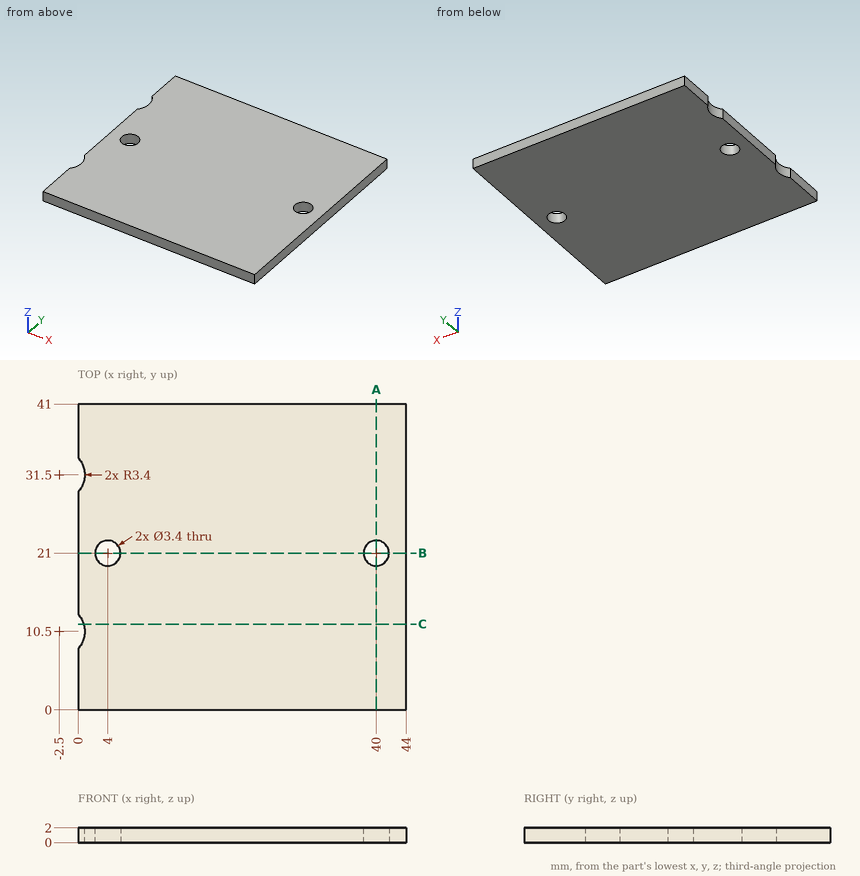
For this review, use the dimensioned drawing (mm, ordinates from the lowest corner) and the shaded views. Give positions to 0.01 mm unless a question says otherwise; leave off trailing zeros. Order: outer loops, then holes, each group sorted by start corner. A loop starts at its lowest first (then second) coordinate and runs counter-clockwise, first axis right, second up.
1. Add section C-C, the plane y = 11.5. State the section outline as (x, z) points.
Solution:
outline: (0.75, 0) - (44, 0) - (44, 2) - (0.75, 2) - close
2. To check wall thickness, follow L1, parallel to Y at x = 40, z = 0.4; L2, parallel to Y at x = 38.5, z = 0.2; L3, parallel to X at y = 33, z = 0.15. State the ranges of each line that lie inside material, in increasing order.
Solution:
L1: y = 0 to 19.3, 22.7 to 41
L2: y = 0 to 20.2, 21.8 to 41
L3: x = 0.55 to 44
3. Add section A-A, the plane x = 40. State the section outline as (y, z) points, then the cut area to 3 significant figures.
Solution:
outline: (0, 0) - (19.3, 0) - (19.3, 2) - (0, 2) - close; (22.7, 0) - (41, 0) - (41, 2) - (22.7, 2) - close
area: 75.2 mm2
4. Add section B-B, the plane y = 21. State the section outline as (x, z) points, then the cut area to 3 significant figures.
Solution:
outline: (0, 0) - (2.3, 0) - (2.3, 2) - (0, 2) - close; (5.7, 0) - (38.3, 0) - (38.3, 2) - (5.7, 2) - close; (41.7, 0) - (44, 0) - (44, 2) - (41.7, 2) - close
area: 74.4 mm2
